Input: part model. Units: mm. Frame: model coordinates. Face numbers are marked on the shaded views. A direction names the side the tool comes from. Coordinates: 2 decimals unless noted, no trailing zeros. Write each loop counter-clockwise with the first axis right and the second up, starting at its lowest first coordinate (ties: lowest second). Pieces come first, ordered by that corner, then holes. Notation, with made-up numbers: (12.25, 55) - (57.25, 55) arc R23 ccw to (57.25, 78) - close; hole circle Ø10 at (16.5, -34.75). An arc over 180 degrees is marked (long way). Use a Markdown table: item, result. Add a question column.
Q1. Section query A-A (x = 5). Return the cut outline in (y, z), then the cut area to 3 significant figures.
Q2. Section query D-D (x = 50). Return the cut outline in (y, z).
Q3. Mould query, pull axis Y, two halves, no side actions, for the marked faces 3, 4 and 5. Classes: released by +Y, released by -Y, zero draft, split by the parting line, or undercut.
Q4. Pin query (flat end, axial travel): P1, Ø5.5, axis at x = 118.5, y = -4.5, coming from the +Z side; P2, Ø6, axis at x = 50, y = 82, coming from the +Z side; P3, Ø3, axis at x = 45, y = 57, coming from the +Z side. Return the tip coordinate at first contact, or that it passes through.
Q5. Material intervals for probe 1 along Y at (x, z) = (109, 1); probe 2 along Y at (x, z) = (-4.5, 33.6); probe 3 along Y at (x, z) = (55, 22.5), sorted ascending. Write a range as from..to.
Q6. Section query C-C (y = 83). Return the cut outline in (x, z).
Q7. Set-up query: the marked faces 1 and 2. Return all of +Z, -Z, +X, -X, +Y, -Y with unobstructed straight access to the full face (end or side cutting, diameter ignored); none if empty.
from build123d import *

# Parameters (mm, degrees)
ESQUISSE1_R             = 2
BOSS_EXTRU_1_DEPTH      = 2
ESQUISSE1_3_W           = 132
ESQUISSE1_3_H           = 106
ESQUISSE1_3_W_2         = 114
ESQUISSE1_3_H_2         = 88
BOSS_EXTRU_2_DEPTH      = 3
ESQUISSE2_W             = 132
ESQUISSE2_H             = 106
BOSS_EXTRU_4_DEPTH      = 32
ENL_V_START             = -5
ESQUISSE3_R             = 3.5
ENL_V_MAT_EXTRU_1_DEPTH = 5
CONG_1_R                = 2


with BuildPart() as part:
    # Esquisse1 → Boss.-Extru.1 (new body)
    with BuildSketch(Plane.XY):
        Polygon((63, 78), (43, 78), (43, 84.300950417), (43, 88), (0, 88), (0, 0), (114, 0), (114, 88), (63, 88), (63, 84.300950417), align=None)
        with Locations((5, 5)):
            Circle(ESQUISSE1_R, mode=Mode.SUBTRACT)
        with Locations((109, 5)):
            Circle(ESQUISSE1_R, mode=Mode.SUBTRACT)
        with Locations((5, 83)):
            Circle(ESQUISSE1_R, mode=Mode.SUBTRACT)
        with Locations((109, 83)):
            Circle(ESQUISSE1_R, mode=Mode.SUBTRACT)
    extrude(amount=BOSS_EXTRU_1_DEPTH)

    # Esquisse1<3> → Boss.-Extru.2 (add)
    with BuildSketch(Plane.XY):
        with Locations((57, 44)):
            Rectangle(ESQUISSE1_3_W, ESQUISSE1_3_H)
        with Locations((57, 44)):
            Rectangle(ESQUISSE1_3_W_2, ESQUISSE1_3_H_2, mode=Mode.SUBTRACT)
    extrude(amount=BOSS_EXTRU_2_DEPTH)

    # Esquisse2 → Boss.-Extru.4 (add)
    with BuildSketch(Plane.XY.offset(3)):
        with Locations((57, 44)):
            Rectangle(ESQUISSE2_W, ESQUISSE2_H)
        with BuildLine():
            Line((-7, -7), (-7, -6.949489743))
            ThreePointArc((-7, -6.949489743), (-6.974873734, -6.974873734), (-6.949489743, -7))
            Line((-6.949489743, -7), (-7, -7))
        make_face(mode=Mode.SUBTRACT)
        Polygon((114, -7), (0, -7), (0, 0), (-7, 0), (-7, 88), (0, 88), (0, 95), (114, 95), (114, 88), (121, 88), (121, 0), (114, 0), align=None, mode=Mode.SUBTRACT)
        with BuildLine():
            ThreePointArc((120.949489743, -7), (120.974873734, -6.974873734), (121, -6.949489743))
            Line((121, -6.949489743), (121, -7))
            Line((121, -7), (120.949489743, -7))
        make_face(mode=Mode.SUBTRACT)
        with BuildLine():
            Line((-7, 95), (-6.949489743, 95))
            ThreePointArc((-6.949489743, 95), (-6.974873734, 94.974873734), (-7, 94.949489743))
            Line((-7, 94.949489743), (-7, 95))
        make_face(mode=Mode.SUBTRACT)
        with BuildLine():
            ThreePointArc((121, 94.949489743), (120.974873734, 94.974873734), (120.949489743, 95))
            Line((120.949489743, 95), (121, 95))
            Line((121, 95), (121, 94.949489743))
        make_face(mode=Mode.SUBTRACT)
    extrude(amount=BOSS_EXTRU_4_DEPTH)

    # Esquisse3 → Enlèv. mat.-Extru.1 (cut)
    with BuildSketch(Plane.XY.offset(35).offset(ENL_V_START)):
        with Locations((-4.5, 92.5)):
            Circle(ESQUISSE3_R)
        with Locations((118.5, 92.5)):
            Circle(ESQUISSE3_R)
        with Locations((118.5, -4.5)):
            Circle(ESQUISSE3_R)
        with Locations((-4.5, -4.5)):
            Circle(ESQUISSE3_R)
    extrude(amount=ENL_V_MAT_EXTRU_1_DEPTH, mode=Mode.SUBTRACT)

    # Congé1
    # the kernel refuses this fillet: 2 mm, written as the material it takes off along each edge
    with BuildSketch(Plane(origin=(114, 88, 3), x_dir=(0, 1, 0), z_dir=(0, 0, 1)), Plane(origin=(114, 0, 3), x_dir=(1, 0, 0), z_dir=(0, 0, 1))) as cong_1_piece_1:
        with BuildLine():
            CenterArc((CONG_1_R, -CONG_1_R), CONG_1_R, 90, 90)
            Line((0, -CONG_1_R), (0, 0))
            Line((0, 0), (CONG_1_R, 0))
        make_face()
    extrude(amount=37, mode=Mode.SUBTRACT)
    with BuildSketch(Plane(origin=(0, 0, 3), x_dir=(-1, 0, 0), z_dir=(0, 0, 1)), Plane(origin=(0, 88, 3), x_dir=(0, 1, 0), z_dir=(0, 0, 1))) as cong_1_piece_2:
        with BuildLine():
            CenterArc((CONG_1_R, CONG_1_R), CONG_1_R, 180, 90)
            Line((0, CONG_1_R), (0, 0))
            Line((0, 0), (CONG_1_R, 0))
        make_face()
    extrude(amount=37, mode=Mode.SUBTRACT)


solid = part.part
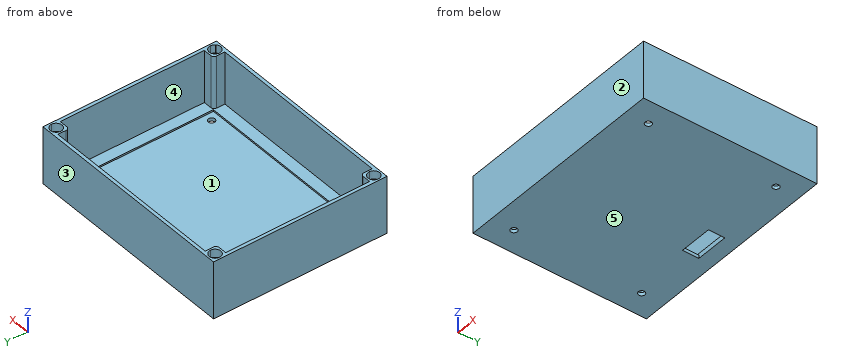
Values follow:
| question | item | result |
|---|---|---|
| 1 | outline | (-9, 0) - (3, 0) - (3, 2) - (0, 2) - (0, 3) - (-7, 3) - (-7, 35) - (-9, 35) - close; (7, 0) - (81, 0) - (81, 2) - (7, 2) - close; (85, 0) - (97, 0) - (97, 35) - (95, 35) - (95, 3) - (88, 3) - (88, 2) - (85, 2) - close |
| 1 | area | 342 mm2 |
| 2 | outline | (-9, 0) - (78, 0) - (78, 2) - (0, 2) - (0, 3) - (-7, 3) - (-7, 35) - (-9, 35) - close; (88, 0) - (97, 0) - (97, 35) - (95, 35) - (95, 3) - (88, 3) - close |
| 3 | face 3 | released by +Y |
| 3 | face 4 | undercut |
| 3 | face 5 | zero draft |
| 4 | P1 | z = 30 |
| 4 | P2 | through |
| 4 | P3 | z = 2 |
| 5 | probe 1 | -9..3, 7..81, 85..97 |
| 5 | probe 2 | -9..-8, -1..0, 88..89, 96..97 |
| 5 | probe 3 | -9..-7, 95..97 |
| 6 | outline | (-9, 0) - (3, 0) - (3, 2) - (0, 2) - (0, 3) - (-7, 3) - (-7, 35) - (-9, 35) - close; (7, 0) - (43, 0) - (43, 2) - (7, 2) - close; (63, 0) - (107, 0) - (107, 2) - (63, 2) - close; (111, 0) - (123, 0) - (123, 35) - (121, 35) - (121, 3) - (114, 3) - (114, 2) - (111, 2) - close |
| 7 | face 1 | +Z |
| 7 | face 2 | +Z, -Z, +X, -X, -Y |
